from build123d import *

# Parameters (mm, degrees)
SKETCH1_W          = 16
SKETCH1_H          = 1500
SKETCH3_R          = 11
CUT_EXTRUDE1_DEPTH = 32
CUT_EXTRUDE2_START = -400
SKETCH4_R          = 38
CUT_EXTRUDE2_DEPTH = 400


with BuildPart() as part:
    # Sketch1 → Revolve1 (revolve)
    with BuildSketch(Plane.XY, mode=Mode.PRIVATE) as revolve1_sk:
        with Locations((767, 750)):
            Rectangle(SKETCH1_W, SKETCH1_H)
    revolve(revolve1_sk.sketch.rotate(Axis((0, 0, 0), (0, 1, 0)), 90), axis=Axis((0, 0, 0), (0, 1, 0)))

    # Sketch2 → Revolve2 (revolve)
    with BuildSketch(Plane(origin=(0, 0, 0), x_dir=(0, 0, -1), z_dir=(1, 0, 0)), mode=Mode.PRIVATE) as revolve2_sk:
        Polygon((1070, 1238), (737, 1238), (737, 1244), (987, 1244), (1038, 1258.624014674), (1038, 1305), (1070, 1305), align=None)
    revolve(revolve2_sk.sketch.rotate(Axis((0, 1200, -775), (0, 0, -1)), 90), axis=Axis((0, 1200, -775), (0, 0, -1)))

    # Sketch3 → Cut-Extrude1 (cut)
    with BuildSketch(Plane(origin=(0, 0, -1070), x_dir=(-1, 0, 0), z_dir=(0, 0, -1))):
        with Locations((0, 1280)):
            Circle(SKETCH3_R)
        with Locations((0, 1120)):
            Circle(SKETCH3_R)
    extrude(amount=-CUT_EXTRUDE1_DEPTH, mode=Mode.SUBTRACT)

    # Sketch4 → Cut-Extrude2 (cut)
    with BuildSketch(Plane(origin=(0, 0, -1070), x_dir=(-1, 0, 0), z_dir=(0, 0, -1)).offset(CUT_EXTRUDE2_START)):
        with Locations(Location((0, 1200, 0), (0, 0, 180))):
            Circle(SKETCH4_R)
    extrude(amount=CUT_EXTRUDE2_DEPTH, mode=Mode.SUBTRACT)


solid = part.part
Here's how the part is built. I have some questions about the finished solid (model axes, mm). A direction names the side the tool comes from. Coordinates: 2 decimals unless noted, no trailing zeros. Order: outer loops, then holes, each group sorted by start corner. A loop starts at its lowest first (then second) coordinate and runs counter-clockwise, first axis right, second up. Notation, with made-up numbers: M 25.25,28 L 47.25,28 A19 ccw 47.25,52 Z; hole C 84,60 d3. An arc over 180 degrees is marked long. Answer as CSV lines item,"result". Start each with the question number.
1. I want a section at C-C, the plane y = 1200. Write out the boundary of the cut face in (x, z), and give its area (3 significant figures).
2. I want a section at A-A, the plane z = 0. Write out the boundary of the cut face in (x, y).
3. I need wall thicknesses on line 1 (Y direction, x = 0, z = -1050); line 2 (X direction, y = 503, z = 0); line 3 (Y direction, x = 0, z = -753.75). Which ranges of each line are inside material? Lowest first, please. Write a range as [from, to].
4. On a 3-axis mill with a long thin cutter (end or side, diameter ignored), from which of +Z, -Z, +X, -X, +Y, -Y can I reach the whole of each face in a straight line? I mean faces 1 (the flat face through (513, 0, 570)), 2 (the conical face through (-6.27, 1152.245, -1001.524)). Say none if no direction works.
5. I want a section at D-D, the plane z = -854.5. Write out the boundary of the cut face in (x, y), and give its area (3 significant figures).
6. I want a section at B-B, the plane x = -665. Write out the boundary of the cut face in (y, z).
7. We'd pull the mould along Z, two halves only. Please class faces 3 (the flat face through (36, 1213, -737)), 4 (the cylindrical face through (-13.669, 1095.894, -1054.224)), 5 (the flat face through (-1, 1245, -1070)), 6 (the flat face through (-45, 1245, -1038)): released by +Z, released by -Z, zero draft, split by the parting line, or undercut.
8. For pin 1 (12 mm diameter, centred on y = 929, z = 449, fed in from -X); pin 2 (20 mm diameter, centred on x = 0, y = 1120, fed in from -Z); pin 3 (8 mm diameter, centred on y = 462.5, z = -141.5, fed in from +X), each with a flat end and sliding along its axis, tell me the tip position at first contact or that it passes through.
Recorded:
1,outline,"M -105,-1070 L -38,-1070 L -38,-737 L -44,-737 L -44,-757.72 A759 cw long 44,-757.72 L 44,-737 L 38,-737 L 38,-1070 L 105,-1070 L 105,-1038 L 58.62,-1038 L 44,-987 L 44,-773.75 A775 ccw long -44,-773.75 L -44,-987 L -58.62,-1038 L -105,-1038 Z"
1,area,"84,300 mm2"
2,outline,"M -775,0 L -759,0 L -759,1500 L -775,1500 Z; M 759,0 L 775,0 L 775,1500 L 759,1500 Z"
3,line 1,"y = [1095, 1109], [1131, 1162], [1238, 1269], [1291, 1305]"
3,line 2,"x = [-775, -759], [759, 775]"
3,line 3,"y = [1156, 1162], [1238, 1244]"
4,face 1,"+Z, -Z, +X, -X, -Y"
4,face 2,"none"
5,outline,"C 0,1200 d88; hole C 0,1200 d76"
5,area,"1,550 mm2"
6,outline,"M 0,-397.99 L 1500,-397.99 L 1500,-365.86 L 0,-365.86 Z; M 0,365.86 L 1500,365.86 L 1500,397.99 L 0,397.99 Z"
7,face 3,"undercut"
7,face 4,"zero draft"
7,face 5,"released by -Z"
7,face 6,"undercut"
8,pin 1,"stops at x = -635.91"
8,pin 2,"stops at z = -775"
8,pin 3,"stops at x = 762.7"
